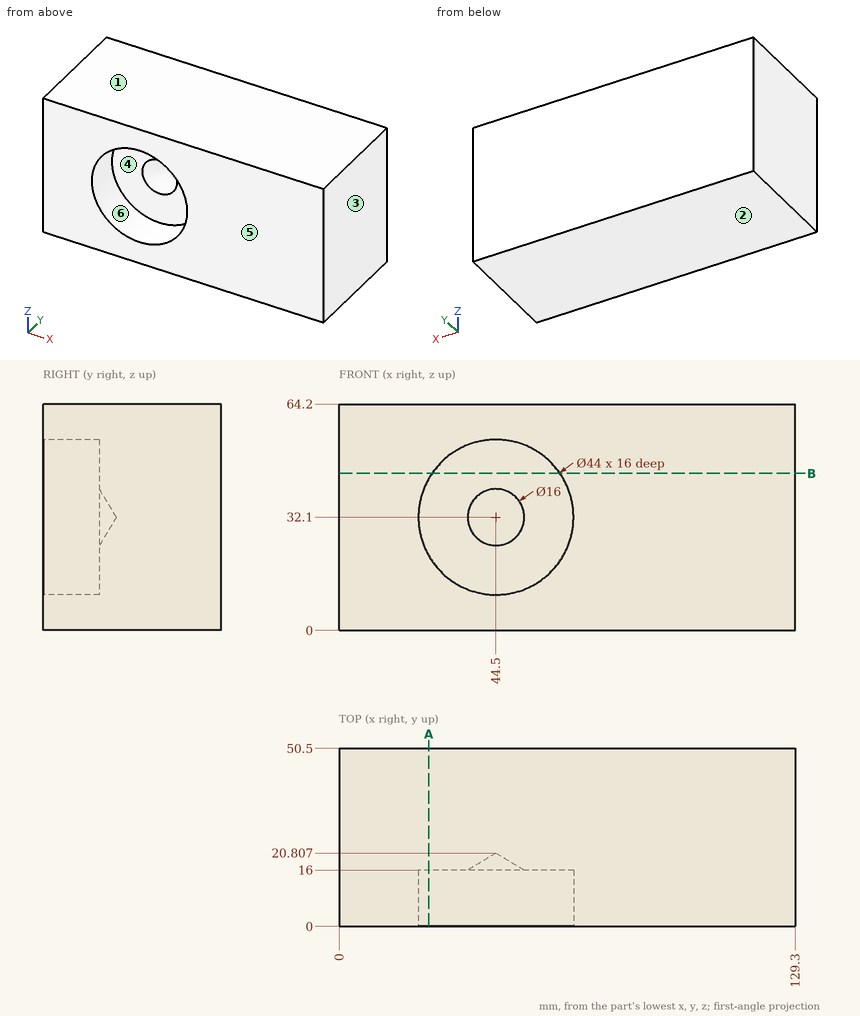
Verification items for this drawing (mm, ordinates from the low corner). A direction names the side the tool comes from. Give positions to 0.01 mm unless a question says otherwise; leave off trailing zeros. Write each loop counter-clockwise with the first axis right and the second up, starting at its lowest first coordinate (ties: lowest second). Pieces come first, ordered by that corner, then holes.
1) Release check for a two-part mould opening along Z. For the marked faces 1, 2, 3 and 4 record: pulls with the +Z half, pulls with the -Z half, needs draft (parallel to the pull), parting line crosses it, or undercut.
2) Gauge pin test, flat end, axial feed: pin 1 (4 mm diameter, centred on y = 15, z = 42.5, fed in from -X). Record the tip position at first contact, or that the pin passes through.
3) Section check A-A, the plane x = 25.5. Record the boundary of the cut face in (y, z).
4) Access from +Z, -Z, +X, -X, +Y, -Y to the whole of each face (thin tool, end or side, straight path). Record for the marked faces 5 and 6.
5) Material ranges on L1, parallel to Z at x = 44.5, y = 12.5; L2, parallel to Z at x = 28, y = 7; L3, parallel to Y at x = 36.5, z = 42, recorded low to high.
6) Section check B-B, the plane z = 44.5. Record the boundary of the cut face in (x, y), and give its area (3 significant figures).
Computed:
1. face 1: pulls with the +Z half
1. face 2: pulls with the -Z half
1. face 3: needs draft
1. face 4: undercut
2. pin 1: stops at x = 0
3. outline: (0, 0) - (50.5, 0) - (50.5, 64.2) - (0, 64.2) - (0, 43.19) - (16, 43.19) - (16, 21.01) - (0, 21.01) - close
4. face 5: +Z, -Z, +X, -X, -Y
4. face 6: -Y
5. L1: z = 0 to 10.1, 54.1 to 64.2
5. L2: z = 0 to 17.55, 46.65 to 64.2
5. L3: y = 16 to 50.5
6. outline: (0, 0) - (26.33, 0) - (26.33, 16) - (62.67, 16) - (62.67, 0) - (129.3, 0) - (129.3, 50.5) - (0, 50.5) - close
6. area: 5,950 mm2
